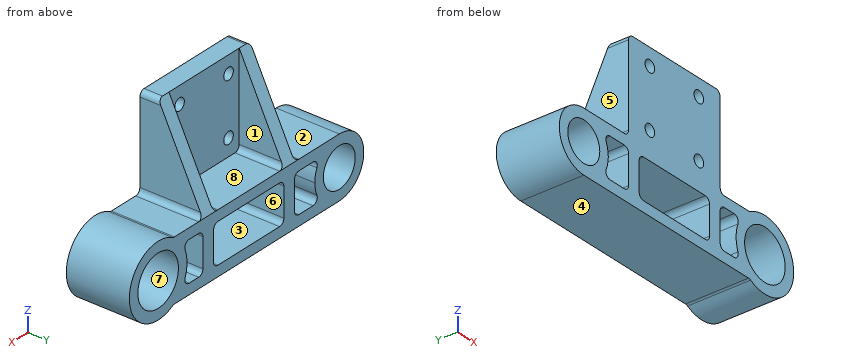
from build123d import *

# Parameters (mm, degrees)
SKETCH1_R               = 7.5
SKETCH1_R_2             = 9.525
BOSS_EXTRUDE1_DEPTH     = 24
SKETCH8_W               = 5
SKETCH8_H               = 17
BOSS_EXTRUDE4_DEPTH     = 35
CUT_EXTRUDE4_DEPTH      = 33.5125
CUT_EXTRUDE4_DEPTH_BACK = 52
SKETCH10_W              = 33
SKETCH10_H              = 15
CUT_EXTRUDE5_DEPTH      = 35
FILLET1_R               = 2
SKETCH12_R              = 2.25
CUT_EXTRUDE6_DEPTH      = 35


with BuildPart() as part:
    # Sketch1 → Boss-Extrude1 (new body)
    with BuildSketch(Plane(origin=(0, 0, 0), x_dir=(1, 0, 0), z_dir=(0, 1, 0))):
        with BuildLine():
            Line((35.393818591, 11.5), (-42.5125, 11.5))
            ThreePointArc((-42.5125, 11.5), (-54.0125, 0), (-42.5125, -11.5))
            Line((-42.5125, -11.5), (35.393818591, -11.5))
            ThreePointArc((35.393818591, -11.5), (56.0375, 0), (35.393818591, 11.5))
        make_face()
        with Locations((-42.5125, 0)):
            Circle(SKETCH1_R, mode=Mode.SUBTRACT)
        with Locations((42.5125, 0)):
            Circle(SKETCH1_R_2, mode=Mode.SUBTRACT)
    extrude(amount=BOSS_EXTRUDE1_DEPTH)

    # Sketch8 → Boss-Extrude4 (add)
    with BuildSketch(Plane.XY.offset(11.5)):
        with Locations((-19, 15.5)):
            Rectangle(SKETCH8_W, SKETCH8_H)
        Polygon((-16.5, 7), (-21.5, 7), (-21.5, 0), (21.5, 0), (21.5, 7), (16.5, 7), align=None)
        with Locations((19, 15.5)):
            Rectangle(SKETCH8_W, SKETCH8_H)
    extrude(amount=BOSS_EXTRUDE4_DEPTH)

    # Sketch9 → Cut-Extrude4 (cut, two sides)
    with BuildSketch(Plane.ZY.offset(21.5)) as cut_extrude4_sk:
        Polygon((11.5, 24), (46.5, 7), (46.5, 24), align=None)
    extrude(amount=CUT_EXTRUDE4_DEPTH, mode=Mode.SUBTRACT)
    extrude(cut_extrude4_sk.sketch, amount=-CUT_EXTRUDE4_DEPTH_BACK, mode=Mode.SUBTRACT)

    # Sketch10 → Cut-Extrude5 (cut)
    with BuildSketch(Plane(origin=(0, 24, 0), x_dir=(1, 0, 0), z_dir=(0, 1, 0))):
        with BuildLine():
            Line((-21.5, 7.5), (-33.794702113, 7.5))
            ThreePointArc((-33.794702113, 7.5), (-31.730462259, 3.999707758), (-31.0125, 0))
            ThreePointArc((-31.0125, 0), (-31.730462259, -3.999707758), (-33.794702113, -7.5))
            Line((-33.794702113, -7.5), (-21.5, -7.5))
            Line((-21.5, -7.5), (-21.5, 7.5))
        make_face()
        Rectangle(SKETCH10_W, SKETCH10_H)
        with BuildLine():
            Line((31.257473345, 7.5), (21.5, 7.5))
            Line((21.5, 7.5), (21.5, -7.5))
            Line((21.5, -7.5), (31.257473345, -7.5))
            ThreePointArc((31.257473345, -7.5), (28.9875, 0), (31.257473345, 7.5))
        make_face()
    extrude(amount=-CUT_EXTRUDE5_DEPTH, mode=Mode.SUBTRACT)

    # Fillet1
    fillet1_edges = [part.edges().sort_by_distance(p)[0] for p in [
        (-16.5, 12, -7.5),
        (16.5, 12, -7.5),
        (31.257473345, 12, -7.5),
        (31.257473345, 12, 7.5),
        (21.5, 12, 7.5),
        (35.393818591, 12, 11.5),
        (21.5, 12, -7.5),
        (35.393818591, 12, -11.5),
        (-21.5, 3.5, 46.5),
        (-16.5, 15.5, 11.5),
        (-21.5, 12, 11.5),
        (16.5, 15.5, 11.5),
        (21.5, 12, 11.5),
        (21.5, 3.5, 46.5),
        (-33.794702113, 12, 7.5),
        (-33.794702113, 12, -7.5),
        (-21.5, 12, -7.5),
        (-21.5, 12, 7.5),
        (16.5, 12, 7.5),
        (-16.5, 12, 7.5),
    ]]
    fillet(fillet1_edges, radius=FILLET1_R)

    # Sketch12 → Cut-Extrude6 (cut)
    with BuildSketch(Plane.XZ):
        with Locations((-11.5, 40)):
            Circle(SKETCH12_R)
        with Locations((-11.5, 18)):
            Circle(SKETCH12_R)
        with Locations((11.5, 40)):
            Circle(SKETCH12_R)
        with Locations((11.5, 18)):
            Circle(SKETCH12_R)
    extrude(amount=-CUT_EXTRUDE6_DEPTH, mode=Mode.SUBTRACT)


solid = part.part
Check sheet for the modelled part. Datum: model origin and axes. Units: mm. Face numbers are marked on the shaded views. A direction names the side the tool comes from. Give positions to 0.01 mm unless a question says otherwise; leave off trailing zeros. Loops run counter-clockwise (first coordinate to the right, second up) from the corner with the lowest first, then second, coordinate; pieces in that order, holes last. Notation, with made-up numbers: M -3.75,16.5 L 27.25,16.5 A30 ccw 27.25,39.5 Z; hole C 65,86 d10. An arc over 180 degrees is marked long. Use a Markdown table: item, result. Add a question column.
Q1. Mould release check, pull along Z, two halves, no side actions. Record for the marked faces 5, 6, 7 and 8: pulls with the +Z half, pulls with the -Z half, needs draft (parallel to the pull), parting line crosses it, or undercut.
Q2. Sectioned sample at C-C, the plane z = 18. Record the cut outline in (x, y), then the cut area to 3 significant figures.
Q3. Tool access check on the marked faces 1, 2, 3 and 4. Record the directions out of +Z, -Z, +X, -X, +Y, -Y that give a thin tool (end or side, any length) a straight path to the whole face; none if there is none.
Q4. Sectioned sample at B-B, the plane x = 26. Record the cut outline in (y, z).
Q5. Scan lines: line 1 along Z through (x, y) = (11.5, 3.25); line 2 along X through (y, z) = (19.5, 3); line 3 along X through (y, z) = (2, 6). Record each from-to range of solid material in increasing order. Write a range as [from, to].
Q6. Sectioned sample at D-D, the plane z = 2. Record the cut outline in (x, y).
Q7. Sectioned sample at A-A, the plane x = -11.5. Record the cut outline in (y, z), then the cut area to 3 significant figures.
Q8. Go/stop test with flat-tipped pins: pin 1 (4 mm diameter, centred on y = 9, z = 32.5, fed in from -X); pin 2 (8 mm diameter, centred on y = 13, z = 29, fed in from +X); pin 3 (9 mm diameter, centred on y = 16.5, z = 1, fed in from +X); pin 4 (7 mm diameter, centred on x = 4.5, y = 15, fed in from -Z). Record where each tip stops, or that it passes through.
Verdict:
| question | item | result |
|---|---|---|
| 1 | face 5 | needs draft |
| 1 | face 6 | undercut |
| 1 | face 7 | undercut |
| 1 | face 8 | pulls with the +Z half |
| 2 | outline | M -21.5,0 L -13.75,0 L -13.75,7 L -16.5,7 L -16.5,20.84 L -21.5,20.84 Z; M -9.25,0 L 9.25,0 L 9.25,7 L -9.25,7 Z; M 13.75,0 L 21.5,0 L 21.5,20.84 L 16.5,20.84 L 16.5,7 L 13.75,7 Z |
| 2 | area | 376 mm^2 |
| 3 | face 1 | +Z, +Y |
| 3 | face 2 | +Z, -X, +Y, -Y |
| 3 | face 3 | +Y, -Y |
| 3 | face 4 | -Z, -X, +Y, -Y |
| 4 | outline | M 0,-11.5 L 24,-11.5 L 24,-7.5 L 0,-7.5 Z; M 0,7.5 L 24,7.5 L 24,11.5 L 0,11.5 Z |
| 5 | line 1 | [-11.5, -7.5], [7.5, 15.75], [20.25, 37.75], [42.25, 46.5] |
| 5 | line 2 | [-53.61, -49.39], [-35.64, -31.41], [-21.5, -16.5], [16.5, 21.5], [29.32, 33.47], [51.55, 55.7] |
| 5 | line 3 | [-52.32, -47.01], [-38.01, -32.12], [-21.56, -16.44], [16.44, 21.56], [29.93, 35.11], [49.91, 54.63] |
| 6 | outline | M -53.84,0 L -49.74,0 L -49.74,24 L -53.84,24 Z; M -35.28,0 L -31.19,0 L -31.19,24 L -35.28,24 Z; M -21.5,0 L -16.5,0 L -16.5,24 L -21.5,24 Z; M 16.5,0 L 21.5,0 L 21.5,24 L 16.5,24 Z; M 29.14,0 L 33.2,0 L 33.2,24 L 29.14,24 Z; M 51.83,0 L 55.89,0 L 55.89,24 L 51.83,24 Z |
| 7 | outline | M 0,-11.5 L 24,-11.5 L 24,-7.5 L 0,-7.5 Z; M 0,7.5 L 24,7.5 L 24,11.5 L 7,11.5 L 7,15.75 L 0,15.75 Z; M 0,20.25 L 7,20.25 L 7,37.75 L 0,37.75 Z; M 0,42.25 L 7,42.25 L 7,46.5 L 0,46.5 Z |
| 7 | area | 374 mm^2 |
| 8 | pin 1 | x = -21.5 |
| 8 | pin 2 | x = 21.5 |
| 8 | pin 3 | x = 56.04 |
| 8 | pin 4 | z = -11.5 |
